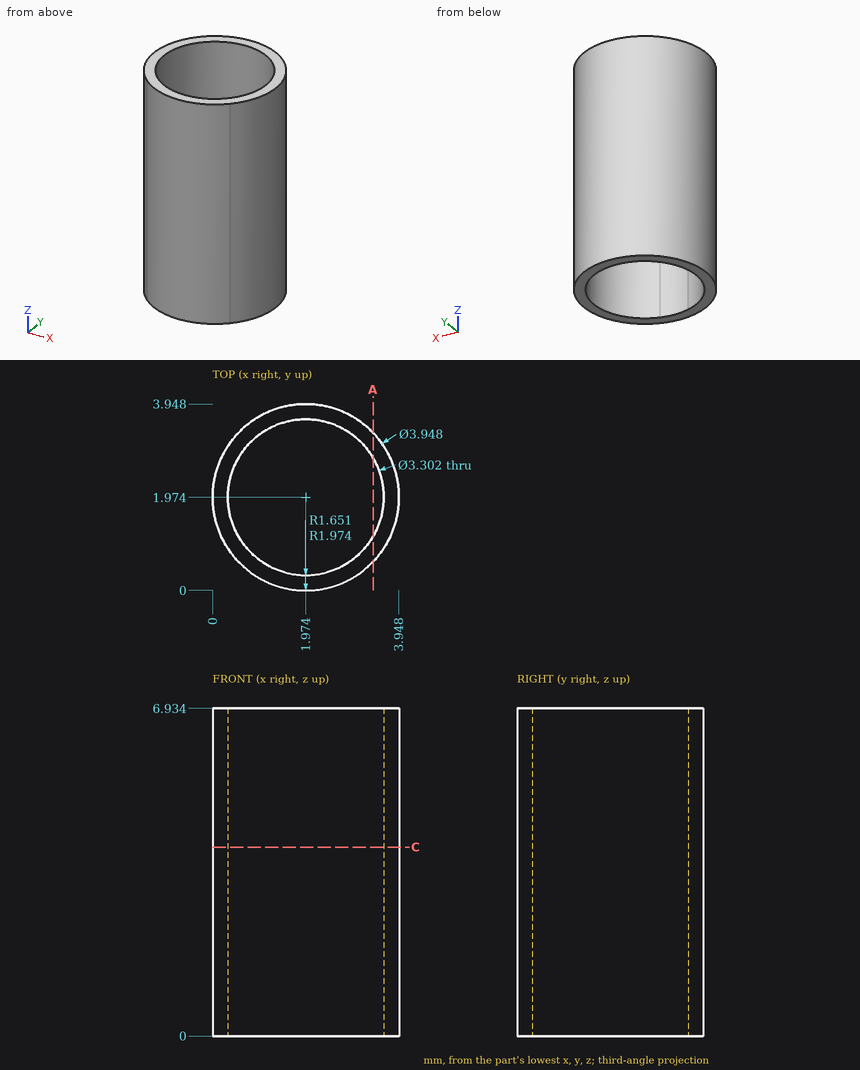
For this review, use the dimensioned drawing (mm, ordinates from the lowest corner) and the shaded views. Round coordinates to 2 decimals unless told otherwise and drop trailing zeros. Order: outer loops, then holes, each group sorted by start corner. A loop starts at its lowest first (then second) coordinate and runs counter-clockwise, first axis right, second up. Notation, with made-up numbers: (29.5, 48.5) -> (44.5, 48.5) arc R17 cw to (44.5, 53.5) -> close; hole circle Ø2 at (-37, 78.5). An arc over 180 degrees is marked (long way). Put each result on its own line as item: value.
Q1. For probe 1 along Y at (x, z) = (1.9, 1) (1 decimal); probe 2 along Y at (x, z) = (0.7, 4) (1 decimal); probe 3 along X at (y, z) = (3.4, 5) (1 decimal), list the stretches that pass through material, from the lowest coordinate up. Write a range as [from, to].
Check result:
probe 1: [0, 0.3], [3.6, 3.9]
probe 2: [0.5, 0.9], [3, 3.5]
probe 3: [0.6, 1.1], [2.8, 3.3]
Q2. Insertion check: pin 1 Ø1.5 at (x, z) = (2.5, 4.5) entering from +Y. The pin has a flat end and moves straight along its axis. Give the tip position at first contact, or say it passes through.
Check result:
pin 1: y = 3.95
Q3. Add section A-A on x = 3.4. Write out the cut boundary in (y, z) (1 decimal).
Check result:
outline: (0.6, 0) -> (1.1, 0) -> (1.1, 6.9) -> (0.6, 6.9) -> close; (2.8, 0) -> (3.3, 0) -> (3.3, 6.9) -> (2.8, 6.9) -> close
Q4. Add section C-C on z = 4. Write out the cut boundary in (x, y) (1 decimal).
Check result:
outline: circle Ø3.9 at (2, 2); hole circle Ø3.3 at (2, 2)
